```python
from build123d import *
from build123d.topology import SkipClean

# Parameters (mm, degrees)
SKETCH1_R           = 19
SKETCH1_R_2         = 2
BOSS_EXTRUDE1_DEPTH = 0.5
SKETCH2_R           = 10
BOSS_EXTRUDE2_DEPTH = 10


with BuildPart() as part:
    # Sketch1 → Boss-Extrude1 (new, symmetric)
    with BuildSketch(Plane(origin=(0, 0, 0), x_dir=(1, 0, 0), z_dir=(0, 1, 0))):
        with Locations(Location((0, 0, 0), (0, 0, 270))):
            Circle(SKETCH1_R)
        with Locations(Location((-14, 0, 0), (0, 0, 270))):
            Circle(SKETCH1_R_2, mode=Mode.SUBTRACT)
        with Locations(Location((7, 12.124355653, 0), (0, 0, 270))):
            Circle(SKETCH1_R_2, mode=Mode.SUBTRACT)
        with Locations(Location((7, -12.124355653, 0), (0, 0, 270))):
            Circle(SKETCH1_R_2, mode=Mode.SUBTRACT)
    extrude(amount=BOSS_EXTRUDE1_DEPTH, both=True)

    # Sketch2 → Boss-Extrude2 (add)
    with BuildSketch(Plane(origin=(0, 0.5, 0), x_dir=(1, 0, 0), z_dir=(0, 1, 0))):
        with Locations(Location((0, 0, 0), (0, 0, 270))):
            Circle(SKETCH2_R)
    extrude(amount=BOSS_EXTRUDE2_DEPTH)

    # Sketch3 → Revolve1 (revolve)
    with SkipClean():  # the faces are left unmerged after this step: merging them gives an invalid solid
        with BuildSketch(Plane(origin=(0, 10.5, 0), x_dir=(1, 0, 0), z_dir=(0, 1, 0))):
            with BuildLine():
                ThreePointArc((9, 0), (6.363961031, 6.363961031), (0, 9))
                Line((0, 9), (0, -9))
                ThreePointArc((0, -9), (6.363961031, -6.363961031), (9, 0))
            make_face()
            with BuildLine():
                Line((0, -9), (0, 9))
                ThreePointArc((0, 9), (-9, 0), (0, -9))
            make_face()
        revolve(axis=Axis((0, 10.5, -9), (0, 0, 1)))


solid = part.part
```
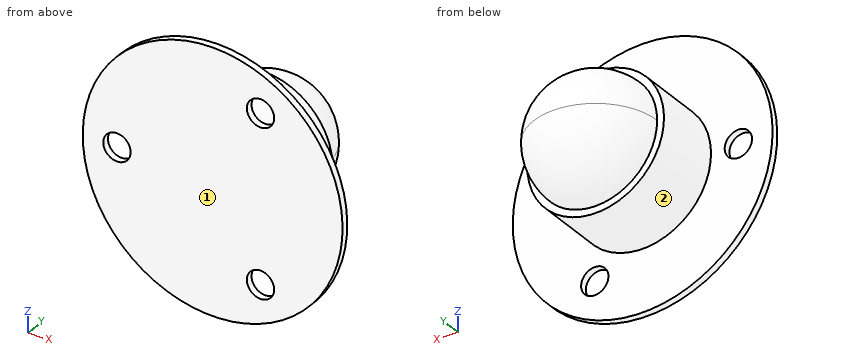
Source: CAD feature listing. Evaluate the final solid. Frame: model axes, mm. Face numbers are marked on the shaded views. A direction names the side the tool comes from. Give positions to 0.01 mm unless a question says otherwise; leave off trailing zeros. Write each loop counter-clockwise with the first axis right and the second up, starting at its lowest first coordinate (ties: lowest second). Pieces come first, ordered by that corner, then holes. Notation, with made-up numbers: (-37, -25.75) - (19, -25.75) arc R17 cw to (19, 1.25) - close; hole circle Ø5 at (14, 63.5). An arc over 180 degrees is marked (long way). One line per item, written item: value. Start each with the question number.
Q1. Set-up query: the marked faces 1 and 2. Return all of +Z, -Z, +X, -X, +Y, -Y with unobstructed straight access to the full face (end or side cutting, diameter ignored); none if empty.
Q2. Section query D-D, the plane y = 3.5. Return the cut outline in (x, z), then the cut area to 3 significant figures.
Q3. Section query C-C, the plane z = 8. Return the cut outline in (x, y).
Q4. First-contact query: pin 1 Ø6 at (y, z) = (6.5, -5) entering from +X; pin 2 Ø2.5 at (x, z) = (-14, 0) entering from -Y; pin 3 Ø6.5 at (x, z) = (7, 12.12) entering from -Y; pin 4 Ø5 at (x, z) = (9, -0.5) entering from +Y. Flat tips, straight axial feed; report the tip coordinate or a pass-through.
Q5. Section query A-A, the plane x = 7. Return the cut outline in (y, z), then the cut area to 3 significant figures.
Q6. Section query B-B, the plane x = -14.5. Return the cut outline in (y, z), then the cut area to 3 significant figures.
Q7. Material intervals for probe 1 along X at (y, z) = (0.35, 0); probe 2 along Y at (x, z) = (4, 10); probe 3 along Y at (x, z) = (-7.5, -5.5), sorted ascending. Write a range as from..to.
Answer:
1. face 1: +Z, -Z, +X, -X, -Y
1. face 2: +Y
2. outline: circle Ø20 at (0, 0)
2. area: 314 mm2
3. outline: (-17.23, -0.5) - (17.23, -0.5) - (17.23, 0.5) - (6, 0.5) - (6, 10.5) - (4.12, 10.5) arc R4.12 ccw to (-4.12, 10.5) - (-6, 10.5) - (-6, 0.5) - (-17.23, 0.5) - close
4. pin 1: stops at x = 9.8
4. pin 2: passes through
4. pin 3: stops at y = -0.5
4. pin 4: stops at y = 16.71
5. outline: (-0.5, -17.66) - (0.5, -17.66) - (0.5, -14.12) - (-0.5, -14.12) - close; (-0.5, -10.12) - (0.5, -10.12) - (0.5, -7.14) - (10.5, -7.14) - (10.5, -5.66) arc R5.66 ccw to (10.5, 5.66) - (10.5, 7.14) - (0.5, 7.14) - (0.5, 10.12) - (-0.5, 10.12) - close; (-0.5, 14.12) - (0.5, 14.12) - (0.5, 17.66) - (-0.5, 17.66) - close
5. area: 220 mm2
6. outline: (-0.5, -12.28) - (0.5, -12.28) - (0.5, -1.94) - (-0.5, -1.94) - close; (-0.5, 1.94) - (0.5, 1.94) - (0.5, 12.28) - (-0.5, 12.28) - close
6. area: 20.7 mm2
7. probe 1: x = -19..-16, -12..19
7. probe 2: y = -0.5..0.5
7. probe 3: y = -0.5..10.5
